The model under review builds one solid part; all positions refer to its coordinate system, in mm. A direction names the side the tool comes from. Round coordinates to 2 decimals unless told otherwise and drop trailing zeros. Write each loop counter-clockwise with the first axis right and the second up, starting at its lowest first coordinate (ties: lowest second). Pieces come first, ordered by that corner, then holes.
Item 1: Add section A-A (y = -39.6). Give the boundary of the cut face in (x, z), plus the area to 3 significant figures.
Item 2: Add section B-B (x = 79). Give the boundary of the cut face in (y, z).
Item 3: Draft analysis for pull direction X (two halves, no side actions). For faces 4 (the face through (48, -8, -3)), 5 (the face through (9.85, -21, -3)), 6 (the face through (8.42, -8.6, -3.45)), state which applies: +X half, -X half, draft (parallel to the pull), parting line (faces both ways), or undercut.
Item 4: Clearance check with flat-ended pins moving along their axes: pin 1 Ø4 at (x, y) = (39, -21) entering from -Z; pin 2 Ø6.5 at (x, z) = (8, -6) entering from +Y; pin 3 Ø8.5 at (x, y) = (56.25, -39.6) entering from +Z; pin 4 Ø2 at (x, z) = (43.5, -4) entering from +Y. State where each tip first meets the part, or that it passes through.
Item 5: To check wall thickness, follow L1, parallel to X at y = -4.7, z = -6.2; L2, parallel to Y at x = 85, z = -5.5; L3, parallel to Y at x = 35, z = -6.25. State the ranges of each line that lie inside material, in increasing order.
Item 6: Add section C-C (y = -19.5). Give the boundary of the cut face in (x, z).
Item 7: Machinability: for faces 1 (the face through (88.58, -32.7, -3.45)), 2 (the face through (49, -33.3, -3)), 3 (the face through (12.5, -4, -4)), which of the approach directions +Z, -Z, +X, -X, +Y, -Y give a long, thin tool a straight path to every point of the face, cutting with its end or side? Answer none if there is none.
```python
from build123d import *

# Parameters (mm, degrees)
SKETCH1_W            = 97
SKETCH1_H            = 51
SKETCH1_R            = 1.6
BOSS_EXTRUDE1_DEPTH  = 1.8
FILLET1_R            = 2
SKETCH4_W            = 8
SKETCH4_H            = 10
SKETCH4_R            = 2
BOSS_EXTRUDE3_DEPTH  = 4
FILLET2_R            = 2
FILLET2_OF_MIRROR1_R = 2
BOSS_EXTRUDE4_DEPTH  = 7
SKETCH7_R            = 2.7
CUT_EXTRUDE3_DEPTH   = 111.223590941
CUT_EXTRUDE4_DEPTH   = 111.223590941
FILLET3_R            = 0.6
CHAMFER1_SIZE        = 1
SKETCH9_W            = 97
SKETCH9_H            = 51
CUT_EXTRUDE5_DEPTH   = 111.223590941


with BuildPart() as part:
    # Sketch1 → Boss-Extrude1 (new body)
    with BuildSketch(Plane.XY):
        with Locations((48.5, -25.5)):
            Rectangle(SKETCH1_W, SKETCH1_H)
        with Locations((92.5, -44.5)):
            Circle(SKETCH1_R, mode=Mode.SUBTRACT)
        with Locations((4.5, -44.5)):
            Circle(SKETCH1_R, mode=Mode.SUBTRACT)
    extrude(amount=BOSS_EXTRUDE1_DEPTH)

    # Fillet1
    fillet1_edges = [part.edges().sort_by_distance(p)[0] for p in [
        (0, 0, 0.9),
        (97, 0, 0.9),
        (97, -51, 0.9),
        (0, -51, 0.9),
    ]]
    fillet(fillet1_edges, radius=FILLET1_R)

    # Sketch4 → Boss-Extrude3 (add)
    with BuildSketch(Plane(origin=(0, -2.5, 0), x_dir=(1, 0, 0), z_dir=(0, 1, 0))):
        with Locations((88.5, 5)):
            Rectangle(SKETCH4_W, SKETCH4_H)
        with Locations(Location((88.5, 6.2, 0), (0, 0, 270))):
            Circle(SKETCH4_R, mode=Mode.SUBTRACT)
    boss_extrude3 = extrude(amount=-BOSS_EXTRUDE3_DEPTH)

    # Fillet2
    fillet2_edges = [part.edges().sort_by_distance(p)[0] for p in [
        (84.5, -4.5, -10),
        (92.5, -4.5, -10),
    ]]
    fillet(fillet2_edges, radius=FILLET2_R)

    # Mirror1: Boss-Extrude3 across plane
    add(boss_extrude3.mirror(Plane(origin=(48.5, 0, 0), x_dir=(0, 0, 1), z_dir=(1, 0, 0))))

    # Fillet2 of Mirror1
    fillet2_of_mirror1_edges = [part.edges().sort_by_distance(p)[0] for p in [
        (12.5, -4.5, -10),
        (4.5, -4.5, -10),
    ]]
    fillet(fillet2_of_mirror1_edges, radius=FILLET2_OF_MIRROR1_R)

    # Sketch5 → Boss-Extrude4 (add)
    with BuildSketch(Plane(origin=(0, 0, 0), x_dir=(-1, 0, 0), z_dir=(0, 0, -1))):
        with BuildLine():
            Line((-89.15, -10), (-89.15, -31.3))
            ThreePointArc((-89.15, -31.3), (-88.564213562, -32.714213562), (-87.15, -33.3))
            Line((-87.15, -33.3), (-9.85, -33.3))
            ThreePointArc((-9.85, -33.3), (-8.435786438, -32.714213562), (-7.85, -31.3))
            Line((-7.85, -31.3), (-7.85, -10))
            ThreePointArc((-7.85, -10), (-8.435786438, -8.585786438), (-9.85, -8))
            Line((-9.85, -8), (-87.15, -8))
            ThreePointArc((-87.15, -8), (-88.564213562, -8.585786438), (-89.15, -10))
        make_face()
        with BuildLine():
            Line((-86.65, -10), (-10.35, -10))
            ThreePointArc((-10.35, -10), (-9.496446609, -9.646446609), (-9.85, -10.5))
            Line((-9.85, -10.5), (-9.85, -30.8))
            ThreePointArc((-9.85, -30.8), (-9.496446609, -31.653553391), (-10.35, -31.3))
            Line((-10.35, -31.3), (-86.65, -31.3))
            ThreePointArc((-86.65, -31.3), (-87.503553391, -31.653553391), (-87.15, -30.8))
            Line((-87.15, -30.8), (-87.15, -10.5))
            ThreePointArc((-87.15, -10.5), (-87.503553391, -9.646446609), (-86.65, -10))
        make_face(mode=Mode.SUBTRACT)
    extrude(amount=BOSS_EXTRUDE4_DEPTH)

    # Sketch7 → Cut-Extrude3 (cut, through all)
    with BuildSketch(Plane.XY.offset(1.8)):
        with Locations((56.25, -39.6)):
            Circle(SKETCH7_R)
    extrude(amount=-CUT_EXTRUDE3_DEPTH, mode=Mode.SUBTRACT)

    # Sketch8 → Cut-Extrude4 (cut, through all)
    with BuildSketch(Plane.XY.offset(1.8)):
        with BuildLine():
            Line((16.5, -42.3), (22.1, -42.3))
            ThreePointArc((22.1, -42.3), (24, -44.2), (22.1, -46.1))
            Line((22.1, -46.1), (16.5, -46.1))
            ThreePointArc((16.5, -46.1), (14.6, -44.2), (16.5, -42.3))
        make_face()
    extrude(amount=-CUT_EXTRUDE4_DEPTH, mode=Mode.SUBTRACT)

    # Fillet3
    fillet3_edges = [part.edges().sort_by_distance(p)[0] for p in [
        (53.55, -39.6, 1.8),
        (14.6, -44.2, 1.8),
        (19.3, -46.1, 1.8),
        (24, -44.2, 1.8),
        (19.3, -42.3, 1.8),
    ]]
    fillet(fillet3_edges, radius=FILLET3_R)

    # Chamfer1
    chamfer1_edges = [part.edges().sort_by_distance(p)[0] for p in [
        (90.9, -44.5, 1.8),
        (2.9, -44.5, 1.8),
    ]]
    chamfer(chamfer1_edges, length=CHAMFER1_SIZE)

    # Sketch9 → Cut-Extrude5 (cut, through all)
    with BuildSketch(Plane.XY.offset(1.8)):
        with Locations((48.5, -25.5)):
            Rectangle(SKETCH9_W, SKETCH9_H)
        with BuildLine():
            Line((0.4, -1.8), (0.4, -49.2))
            ThreePointArc((0.4, -49.2), (0.810050506, -50.189949494), (1.8, -50.6))
            Line((1.8, -50.6), (95.2, -50.6))
            ThreePointArc((95.2, -50.6), (96.189949494, -50.189949494), (96.6, -49.2))
            Line((96.6, -49.2), (96.6, -1.8))
            ThreePointArc((96.6, -1.8), (96.189949494, -0.810050506), (95.2, -0.4))
            Line((95.2, -0.4), (1.8, -0.4))
            ThreePointArc((1.8, -0.4), (0.810050506, -0.810050506), (0.4, -1.8))
        make_face(mode=Mode.SUBTRACT)
    extrude(amount=-CUT_EXTRUDE5_DEPTH, mode=Mode.SUBTRACT)


solid = part.part
```
Numbers:
1. outline: (0.4, 0) - (53.55, 0) - (53.55, 1.2) arc R0.6 ccw to (52.95, 1.8) - (0.4, 1.8) - close; (58.95, 0) - (96.6, 0) - (96.6, 1.8) - (59.55, 1.8) arc R0.6 ccw to (58.95, 1.2) - close
1. area: 163 mm2
2. outline: (-50.6, 0) - (-33.3, 0) - (-33.3, -7) - (-31.3, -7) - (-31.3, 0) - (-10, 0) - (-10, -7) - (-8, -7) - (-8, 0) - (-0.4, 0) - (-0.4, 1.8) - (-50.6, 1.8) - close
3. face 4: draft
3. face 5: undercut
3. face 6: -X half
4. pin 1: stops at z = 0
4. pin 2: stops at y = -2.5
4. pin 3: stops at z = 1.8
4. pin 4: stops at y = -8
5. L1: x = 4.5 to 6.5, 10.5 to 12.5, 84.5 to 86.5, 90.5 to 92.5
5. L2: y = -33.3 to -31.3, -10 to -8, -6.5 to -2.5
5. L3: y = -33.3 to -31.3, -10 to -8
6. outline: (0.4, 0) - (7.85, 0) - (7.85, -7) - (9.85, -7) - (9.85, 0) - (87.15, 0) - (87.15, -7) - (89.15, -7) - (89.15, 0) - (96.6, 0) - (96.6, 1.8) - (0.4, 1.8) - close
7. face 1: -Z, +X, -Y
7. face 2: -Z, +X, -X, -Y
7. face 3: -Z, +Y
